Can you work these out from the model? Positions are in its coordinate system, mm. A direction names the side the tool comes from. Round coordinates to 2 decimals unless told otherwise and drop trailing zeros. Loops run counter-clockwise (first coordinate to the right, second up) from the corner with the lowest first, then second, coordinate; pieces in that order, holes last. Notation, with made-up numbers: (71.25, 79.25) -> (112.25, 79.25) arc R9 ccw to (112.25, 95.25) -> close; hole circle Ø6 at (-39.75, -27.75). An arc over 180 degrees is marked (long way). Use a Markdown table: item, result.
from build123d import *

# Parameters (mm, degrees)
BOSS_EXTRUDE1_DEPTH = 50
SKETCH3_W           = 66.376369139
SKETCH3_H           = 188.96079622
CUT_EXTRUDE1_DEPTH  = 305.408240944
SKETCH4_R           = 34.5
CUT_EXTRUDE2_DEPTH  = 13


with BuildPart() as part:
    # Sketch1 → Boss-Extrude1 (new body)
    with BuildSketch(Plane.XY):
        with BuildLine():
            Line((0.221790001, 84.828286355), (0.2207262, 284.828286352))
            add(Edge.make_bspline(
                [(0.2207262, 284.828286352), (-159.978737061, 262.606607754), (-63.000724603, 150.139017081), (-35, 85.625)],
                knots=[0, 0, 0, 0, 1, 1, 1, 1], degree=3))
            Line((-35, 85.625), (-35, -85.625))
            Line((-35, -85.625), (35, -85.625))
            Line((35, -85.625), (35, -40.1019375))
            Line((35, -40.1019375), (0.221790001, 84.828286355))
        make_face()
    extrude(amount=BOSS_EXTRUDE1_DEPTH)

    # Sketch3 → Cut-Extrude1 (cut, through all)
    with BuildSketch(Plane(origin=(22.122011617, 6.158349372, 0), x_dir=(0, 0, -1), z_dir=(0.9633678796634119, 0.2681833858254875, 0))):
        with Locations((8.18818457, -12.819032142)):
            Rectangle(SKETCH3_W, SKETCH3_H)
    extrude(amount=-CUT_EXTRUDE1_DEPTH, mode=Mode.SUBTRACT)

    # Sketch4 → Cut-Extrude2 (cut)
    with BuildSketch(Plane(origin=(0, 0, 25), x_dir=(-1, 0, 0), z_dir=(0, 0, -1))):
        Circle(SKETCH4_R)
    extrude(amount=-CUT_EXTRUDE2_DEPTH, mode=Mode.SUBTRACT)


solid = part.part
1. I want a section at A-A (x = 10.5). Please give me the cut outline in (y, z) (3 decimals).
Answer sheet:
| item | result |
|---|---|
| outline | (-85.625, 25) -> (-32.863, 25) -> (-32.863, 38) -> (32.863, 38) -> (32.863, 25) -> (47.907, 25) -> (47.907, 50) -> (-85.625, 50) -> close |
2. I want a section at B-B (y = 14). Please give me the cut outline in (x, z), plus the area to 3 significant figures.
Answer sheet:
| item | result |
|---|---|
| outline | (-35, 25) -> (-31.53, 25) -> (-31.53, 38) -> (19.94, 38) -> (19.94, 50) -> (-35, 50) -> close |
| area | 704 mm² |
3. Will these pins go through, and if not, where does the flat tip stop? pin 1 Ø15 at (y, z) = (19, 27) entering from -X; pin 2 Ø12 at (x, y) = (4.5, 169.5) entering from +Z; pin 3 Ø8 at (y, z) = (195.5, 14) entering from +X; pin 4 Ø10 at (x, z) = (-14, 9.5) entering from -Y.
Answer sheet:
| item | result |
|---|---|
| pin 1 | stops at x = -35 |
| pin 2 | stops at z = 50 |
| pin 3 | stops at x = 0.22 |
| pin 4 | stops at y = 79.48 |
4. Which directions (+Z, -Z, +X, -X, +Y, -Y) give clear straight access to the entire face, cutting with the end or side of a thin tool? Please do faces 1 (the cylindrical face through (-32.92, -10.32, 31.41)), 2 (the flat face through (-27, 100, 50)), 3 (the flat face through (-35, 1, 36)).
Answer sheet:
| item | result |
|---|---|
| face 1 | -Z |
| face 2 | +Z, +X, -X, +Y, -Y |
| face 3 | +Z, -Z, -X, -Y |
5. I need wall thicknesses on line 1 (Y direction, x = 0, z = 30.75) (3 decimals); line 2 (X direction, y = 0, z = 29.5); line 3 (Z direction, x = -10, y = -31). Which ranges of each line are inside material? Lowest first, please.
Answer sheet:
| item | result |
|---|---|
| line 1 | y = -85.625 to -34.5, 34.5 to 284.798 |
| line 2 | x = -35 to -34.5 |
| line 3 | z = 38 to 50 |
6. If we mould it in two halves opening along Y, with no side actions, what happens to faces 4 (the flat face through (-17.143, 79.994, 12.675)), 5 (the flat face through (35, -63, 37)), 6 (the flat face through (-2, 0, 38))? For each: +Y half, -Y half, draft (parallel to the pull), parting line (faces both ways), or undercut.
Answer sheet:
| item | result |
|---|---|
| face 4 | -Y half |
| face 5 | draft |
| face 6 | undercut |
